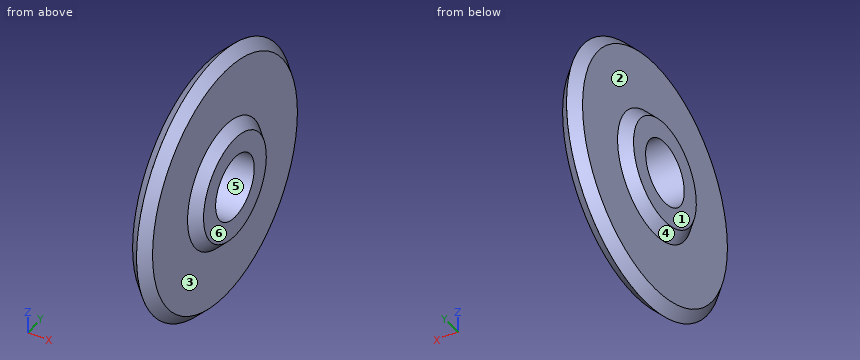
Autodesk Inventor part; units mm, degrees
ref_plane "YZ Plane" through (0, 0, 0) normal (1, 0, 0) x (0, 1, 0)
ref_plane "XZ Plane" through (0, 0, 0) normal (0, 1, 0) x (-1, 0, 0)
ref_plane "XY Plane" through (0, 0, 0) normal (0, 0, 1) x (1, 0, 0)
sketch "Sketch1" plane through (0, 0, 0) normal (0, 1, 0) x (-1, 0, 0)
  line L0 (0, 0) -> (1, 0)
  line L1 (1, 0) -> (1, -6.5)
  line L2 (1, -6.5) -> (0, -6.5)
  line L3 (0, -6.5) -> (0, 0)
  line L4 (1, 0) -> (0, 0)
  line L5 (0, 0) -> (0, -1.6)
  line L6 (0, -1.6) -> (1, -1.6)
  line L7 (1, -1.6) -> (1, 0)
  line L8 (1, -1.6) -> (1.5, -1.6)
  line L9 (1.5, -1.6) -> (1.5, -2.6)
  line L10 (1.5, -2.6) -> (1, -2.6)
  line L11 (1, -2.6) -> (1, -1.6)
  line L12 (0, -1.6) -> (-0.5, -1.6)
  line L13 (-0.5, -1.6) -> (-0.5, -2.6)
  line L14 (-0.5, -2.6) -> (0, -2.6)
  line L15 (0, -2.6) -> (0, -1.6)
  dimension "d0" = 1
  dimension "d1" = 6.5
  dimension "d2" = 1.6
  dimension "d3" = 0.5
  dimension "d4" = 1
  dimension "d5" = 0.5
  dimension "d6" = 1
revolve "Revolution1" add sketch "Sketch1" angle 360 about axis through (0, 0, 0) along (-1, 0, 0) contours L6 L1 L2 L3 | L3 L14 L13 L12 | L8 L9 L10 L1
chamfer "Chamfer1" distance 0.5 angle 45 4 edges at (-1, 0, 2.6) (0, 0, 2.6) (0, 0, 6.5) (-1, 0, 6.5)
properties part number "idler_spacer"
Can you work these out from the model? Positions are in its coordinate system, mm. Face numbers are marked on the shaded views. A direction names the side the tool comes from. Round coordinates to 2 decimals unless told otherwise and drop trailing zeros. Loops run counter-clockwise (first coordinate to the right, second up) from the corner with the lowest first, then second, coordinate; pieces in that order, holes last. Notation, with made-up numbers: M -32.5,-15 L 22.5,-15 A22 ccw 22.5,14 Z; hole C 24,56.5 d2. An arc over 180 degrees is marked long. Answer as a JSON object with one key per item and string values. Group by question number.
Q1. We'd pull the mould along Z, two halves only. Please class the marked faces 4, 5 and 6: +Z half, -Z half, draft (parallel to the pull), parting line (faces both ways), or undercut.
Q2. Please list where these lines run through material, in increasing order: L1, parallel to X at y = 2.5, z = 5.25; L2, parallel to Y at x = -0.65, z = 0; L3, parallel to Z at x = -0.25, y = 1.
Q3. On a 3-axis mill with a long thin cutter (end or side, diameter ignored), from which of +Z, -Z, +X, -X, +Y, -Y can I reach the whole of each face in a straight line? I mean the marked faces 1, 2 and 3. Say none if no direction works.
Q4. Will these pins go through, and if not, where does the flat tip stop? pin 1 (3 mm diameter, centred on y = 0, z = 0, fed in from -X); pin 2 (4 mm diameter, centred on y = 4.5, z = -5, fed in from -X).
Q5. Imagine slicing it at C-C, the plane x = -0.3. Please give me the cut outline in (y, z), then the cut area to 3 significant figures.
Findings:
{
 "1": {"face 4": "parting line", "face 5": "undercut", "face 6": "draft"},
 "2": {"L1": "x = -1 to 0", "L2": "y = -6.35 to -1.6, 1.6 to 6.35", "L3": "z = -6.17 to -1.25, 1.25 to 6.17"},
 "3": {"face 1": "+Z, -Z, -X, +Y, -Y", "face 2": "-X", "face 3": "+X"},
 "4": {"pin 1": "passes through", "pin 2": "stops at x = -1"},
 "5": {"outline": "C 0,0 d12.6; hole C 0,0 d3.2", "area": "117 mm2"}
}
